Could you check a few things on this model? Use its own coordinates, in mm. A direction names the side the tool comes from. Coordinates: 2 decimals unless noted, no trailing zeros. Loops run counter-clockwise (first coordinate to the right, second up) from the corner with the lowest first, then second, coordinate; pieces in that order, holes last. Notation, with made-up numbers: (-14.75, 5.5) -> (16.25, 5.5) arc R18 cw to (16.25, 21.5) -> close; hole circle Ø6 at (53.5, 64). An arc over 180 degrees is marked (long way). One line per question, with ' | ' between items.
```python
from build123d import *
from OCP.BRepFilletAPI import BRepFilletAPI_MakeChamfer

# Parameters (mm, degrees)
SKETCH1_R           = 2.4
BOSS_EXTRUDE1_DEPTH = 0.55
SKETCH2_R           = 1.875
BOSS_EXTRUDE2_DEPTH = 1.65
SKETCH3_R           = 2.5
BOSS_EXTRUDE3_DEPTH = 2
SKETCH4_R           = 2.25
BOSS_EXTRUDE4_DEPTH = 0.8
CUT_EXTRUDE1_REACH  = 8.124
SKETCH5_W           = 0.75
SKETCH5_H           = 6.07376998
CHAMFER1_SIZE       = 0.4
CHAMFER1_SIZE2      = 0.692820323
SKETCH6_W           = 6.999273813
SKETCH6_H           = 5.334981493
SKETCH6_W_2         = 6.558585844
SKETCH6_H_2         = 3.75
CUT_EXTRUDE3_DEPTH  = 2
FILLET2_R           = 1
SKETCH7_R           = 1
CUT_EXTRUDE4_DEPTH  = 2


with BuildPart() as part:
    # Sketch1 → Boss-Extrude1 (new body)
    with BuildSketch(Plane.XY):
        Circle(SKETCH1_R)
    extrude(amount=BOSS_EXTRUDE1_DEPTH)

    # Sketch2 → Boss-Extrude2 (add)
    with BuildSketch(Plane.XY.offset(0.55)):
        Circle(SKETCH2_R)
    extrude(amount=BOSS_EXTRUDE2_DEPTH)

    # Sketch3 → Boss-Extrude3 (add)
    with BuildSketch(Plane(origin=(0, 0, 0), x_dir=(-1, 0, 0), z_dir=(0, 0, -1))):
        Circle(SKETCH3_R)
    extrude(amount=BOSS_EXTRUDE3_DEPTH)

    # Sketch4 → Boss-Extrude4 (add)
    with BuildSketch(Plane.XY.offset(2.2)):
        Circle(SKETCH4_R)
    extrude(amount=BOSS_EXTRUDE4_DEPTH)

    # Cut-Extrude1: up to this face of the body (flat: up to its plane)
    cut_extrude1_end = Plane(part.part.faces().sort_by_distance((-2.332117749, 0, 0.55))[0])
    # Sketch5 → Cut-Extrude1 (cut, up to the picked face)
    with BuildSketch(Plane.XY.offset(3), mode=Mode.PRIVATE) as cut_extrude1_sk1:
        Rectangle(SKETCH5_W, SKETCH5_H)
    cut_extrude1_tool1 = split(extrude(cut_extrude1_sk1.sketch, amount=-CUT_EXTRUDE1_REACH, mode=Mode.PRIVATE), bisect_by=cut_extrude1_end, keep=Keep.BOTH, mode=Mode.PRIVATE)
    add(cut_extrude1_tool1.solids().sort_by(Axis((0, 0, 3), (0, 0, -1)))[0], mode=Mode.SUBTRACT)

    # Chamfer1: one chamfer whose edges measure the first distance from different faces: ONE call of the kernel's chamfer builder (chamfer() names one face for all edges)
    chamfer1_edges_1 = [part.edges().sort_by_distance(p)[0] for p in [
        (-2.25, 0, 3),
    ]]
    chamfer1_side_1 = [part.faces().sort_by_distance(p)[0] for p in [
        (-2.25, 0, 2.6),
    ]]
    chamfer1_edges_2 = [part.edges().sort_by_distance(p)[0] for p in [
        (2.25, 0, 3),
    ]]
    chamfer1_side_2 = [part.faces().sort_by_distance(p)[0] for p in [
        (2.25, 0, 2.6),
    ]]
    chamfer1 = BRepFilletAPI_MakeChamfer(part.part.solid().wrapped)
    for e in chamfer1_edges_1:
        chamfer1.Add(CHAMFER1_SIZE, CHAMFER1_SIZE2, e.wrapped, chamfer1_side_1[0].wrapped)  # the first distance lies on this face
    for e in chamfer1_edges_2:
        chamfer1.Add(CHAMFER1_SIZE, CHAMFER1_SIZE2, e.wrapped, chamfer1_side_2[0].wrapped)  # the first distance lies on this face
    add(Compound.cast(chamfer1.Shape()), mode=Mode.REPLACE)

    # Sketch6 → Cut-Extrude3 (cut)
    with BuildSketch(Plane.XY.offset(3)):
        with Locations((0.047792, -0.043471688)):
            Rectangle(SKETCH6_W, SKETCH6_H)
        Rectangle(SKETCH6_W_2, SKETCH6_H_2, mode=Mode.SUBTRACT)
    extrude(amount=-CUT_EXTRUDE3_DEPTH, mode=Mode.SUBTRACT)

    # Fillet2
    fillet2_edges = [part.edges().sort_by_distance(p)[0] for p in [
        (-1.243734296, 1.875, 2.4),
        (1.243734296, 1.875, 2.4),
        (-1.243734296, -1.875, 2.4),
        (1.243734296, -1.875, 2.4),
    ]]
    fillet(fillet2_edges, radius=FILLET2_R)

    # Sketch7 → Cut-Extrude4 (cut)
    with BuildSketch(Plane(origin=(0, 0, -2), x_dir=(-1, 0, 0), z_dir=(0, 0, -1))):
        Circle(SKETCH7_R)
    extrude(amount=-CUT_EXTRUDE4_DEPTH, mode=Mode.SUBTRACT)


solid = part.part
```
Q1. Imagine slicing it at B-B on x = 0. Write out the boundary of the cut face in (y, z).
Values follow:
outline: (-2.5, -2) -> (-1, -2) -> (-1, 0) -> (1, 0) -> (1, -2) -> (2.5, -2) -> (2.5, 0) -> (2.4, 0) -> (2.4, 0.55) -> (-2.4, 0.55) -> (-2.4, 0) -> (-2.5, 0) -> close
Q2. For pin 1 (0.6 mm diameter, centred on x = 0, y = 0.5, fed in from -Z); pin 2 (2 mm diameter, centred on x = -2, z = 0.5, fed in from -Y); pin 3 (1.2 mm diameter, centred on y = 0.5, z = 2, fed in from +X), each with a flat end and sliding along its axis, tell me the tip position at first contact or that it passes through.
Values follow:
pin 1: stops at z = 0 | pin 2: stops at y = -2.23 | pin 3: stops at x = 2.25
Q3. Please list where these lines run through material, in increasing order: L1, parallel to Y at x = 0, z = -1.15; L2, parallel to Z at x = 0.95, y = -2.1; L3, parallel to Z at x = 0.15, y = -0.3. Write a range as [from, to].
Values follow:
L1: y = [-2.5, -1], [1, 2.5] | L2: z = [-2, 0.55] | L3: z = [0, 0.55]
Q4. Imagine slicing it at A-A on z = 2.45. Write out the boundary of the cut face in (x, y) (3 decimals), plus the area to 3 significant figures.
Values follow:
outline: (-1.607, -1.575) arc R1 ccw to (-0.893, -1.875) -> (-0.375, -1.875) -> (-0.375, 1.875) -> (-0.893, 1.875) arc R1 ccw to (-1.607, 1.575) arc R2.25 ccw to start; (0.375, -1.875) -> (0.893, -1.875) arc R1 ccw to (1.607, -1.575) arc R2.25 ccw to (1.607, 1.575) arc R1 ccw to (0.893, 1.875) -> (0.375, 1.875) -> close | area: 11.8 mm2
Q5. We'd pull the mould along Z, two halves only. Please class faces 1 (the face through (0, 0, 0.55)), 2 (the face through (-1.744, 0.034, 2.892)), 3 (the face through (0, -1, -1)): released by +Z, released by -Z, zero draft, split by the parting line, or undercut.
Values follow:
face 1: undercut | face 2: released by +Z | face 3: zero draft
Q6. Imagine slicing it at C-C on y = 0. Write out the boundary of the cut face in (x, z) (3 decimals), plus the area to 3 significant figures.
Values follow:
outline: (-2.5, -2) -> (-1, -2) -> (-1, 0) -> (1, 0) -> (1, -2) -> (2.5, -2) -> (2.5, 0) -> (2.4, 0) -> (2.4, 0.55) -> (1.875, 0.55) -> (1.875, 2.2) -> (2.25, 2.2) -> (2.25, 2.6) -> (1.557, 3) -> (0.375, 3) -> (0.375, 0.55) -> (-0.375, 0.55) -> (-0.375, 3) -> (-1.557, 3) -> (-2.25, 2.6) -> (-2.25, 2.2) -> (-1.875, 2.2) -> (-1.875, 0.55) -> (-2.4, 0.55) -> (-2.4, 0) -> (-2.5, 0) -> close | area: 16.3 mm2
Q7. For faces 4 (the face through (-0.375, 0, 2)), 5 (the face through (-2.01, 0.29, 2.2)), 6 (the face through (1.875, -0.036, 1.363)), 7 (the face through (0, 0, 0)), 8 (the face through (1.29, 2.024, 0.271)), which set-ups out of +Z, -Z, +X, -X, +Y, -Y let a thin tool reach every point of the face, with its end or its side?
Values follow:
face 4: +Z, +Y, -Y | face 5: -X | face 6: +X | face 7: -Z | face 8: +Z
Q8. Imagine slicing it at D-D on z = 1.9. Write out the boundary of the cut face in (x, y) (3 decimals), plus the area to 3 significant figures.
Values follow:
outline: (-0.375, -1.837) -> (-0.375, 1.837) arc R1.875 ccw to start; (0.375, -1.837) arc R1.875 ccw to (0.375, 1.837) -> close | area: 8.25 mm2
